Autodesk Inventor part; units mm, degrees
ref_plane "YZ Plane" through (0, 0, 0) normal (1, 0, 0) x (0, 1, 0)
ref_plane "XZ Plane" through (0, 0, 0) normal (0, 1, 0) x (-1, 0, 0)
ref_plane "XY Plane" through (0, 0, 0) normal (0, 0, 1) x (1, 0, 0)
sketch "스케치1" plane through (0, 0, 0) normal (0, 0, 1) x (1, 0, 0)
  circle A0 centre (-35.1217, 0) radius 22.9499
  circle A1 centre (-35.1217, 0) radius 11.4294
  line L0 (-20.9226, -18.03) -> (64.9173, -18.03)
  line L1 (64.9173, -18.03) -> (64.9173, 18.03)
  line L2 (64.9173, 18.03) -> (-20.9226, 18.03)
  point P0 (0, 0)
extrude "돌출1" add sketch "스케치1" along normal blind 30 contours A0 L2 L1 L0
extrude "돌출2" add sketch "스케치1" along normal blind 40 contours A0
sketch "스케치2" plane through (-35.1217, 0, 40) normal (0, 0, 1) x (1, 0, 0)
  circle A0 centre (0, 0) radius 11.4294
  line L0 (9.9823, 5.5664) -> (22.2646, 5.5664)
  circle A1 centre (0, 0) radius 22.9499
  line L1 (9.9823, -5.5664) -> (22.2646, -5.5664)
  line L2 (-9.9823, 5.5664) -> (-22.2646, 5.5664)
  line L3 (-9.9823, -5.5664) -> (-22.2646, -5.5664)
  point P0 (35.1217, 0)
extrude "돌출3" add sketch "스케치2" along normal blind 10 contours A0 L0 A1 L1 | A0 L3 A1 L2
sketch "스케치3" plane through (0, 0, 30) normal (0, 0, 1) x (1, 0, 0)
  line L0 (64.9173, -18.03) -> (64.9173, 18.03)
  line L1 (-5.4969, 10.1103) -> (64.9173, 10.1103)
  line L2 (64.9173, 10.1103) -> (64.9173, -11.6809)
  line L3 (64.9173, -11.6809) -> (-5.4969, -11.6809)
  line L4 (-5.4969, -11.6809) -> (-5.4969, 10.1103)
  circle A0 centre (15.1164, 0) radius 4.8497
  circle A1 centre (45.3492, 0) radius 4.9674
  point P0 (0, 0)
extrude "돌출4" cut sketch "스케치3" against normal blind 50 contours A0 | A1
extrude "돌출5" cut sketch "스케치3" against normal blind 20
chamfer "모따기1" distance 13 angle 45 2 edges at (64.9173, 14.0702, 30) (64.9173, -14.8554, 30)
properties part number "240510_3Dsketch06"
Source: CAD feature listing. Evaluate the final solid. Frame: model axes, mm. A direction names the side the tool comes from. Coordinates: 2 decimals unless noted, no trailing zeros. Write each loop counter-clockwise with the first axis right and the second up, starting at its lowest first coordinate (ties: lowest second). Pieces come first, ordered by that corner, then holes. Notation, with made-up numbers: (-17, 89) -> (8, 89) arc R23 ccw to (8, 118) -> close; hole circle Ø4 at (7.25, 46). An arc over 180 degrees is marked (long way). Return JSON: item names as keys, results as strings. Group by question number.
1) Mould query, pull axis Y, two halves, no side actions, for faces 1 (the face through (23, 18.03, 15)), 2 (the face through (-19, 0, 50)), 3 (the face through (-5.497, -1, 20)), 4 (the face through (-57.75, -3.84, 24.65)). Classes: +Y half, -Y half, draft (parallel to the pull), parting line (faces both ways), or undercut.
2) Contact query for flat-ended pins moving along their axis: P1, Ø3, axis at x = -21.5, z = 45, coming from the +Y side; P2, Ø8.5, axis at x = -36.5, y = 11, coming from the +Z side; P3, Ø15, axis at x = 24.5, z = 17.5, coming from the -Y side. Output: stop coordinate, or through.
3) Section query A-A, the plane y = -8. Return loops of the section in (x, z), plus the area to 3 significant figures.
4) Section query C-C, the plane y = -3. Return loops of the section in (x, z), plus the area to 3 significant figures.
5) Ray query, line 1 along Y through (x, z) = (4, 13.5); line 2 along Y through (x, z) = (-7, 23); line 3 along X through (y, z) = (4, 35.5). Return the intervals inside material, ascending.
6) Set-up query: faces 5 (the face through (58.33, 14.13, 23.59)), 6 (the face through (-51, -5.566, 45)), 7 (the face through (29, 10.11, 20)), 8 (the face through (-19, 5.566, 45)). Return all of +Z, -Z, +X, -X, +Y, -Y with unobstructed straight access to the full face (end or side cutting, diameter ignored); none if empty.
7) Section query B-B, the plane z = 8. Return loops of the section in (x, y).
8) Section query D-D, the plane x = 23. Return loops of the section in (y, z), plus the area to 3 significant figures.
From the geometry:
{
 "1": {"face 1": "+Y half", "face 2": "draft", "face 3": "undercut", "face 4": "parting line"},
 "2": {"P1": "y = 5.57", "P2": "z = 40", "P3": "y = -18.03"},
 "3": {"outline": "(-56.63, 0) -> (-43.28, 0) -> (-43.28, 40) -> (-56.63, 40) -> close; (-26.96, 0) -> (64.92, 0) -> (64.92, 10) -> (-5.5, 10) -> (-5.5, 30) -> (-13.61, 30) -> (-13.61, 40) -> (-26.96, 40) -> close", "area": "2,020 mm²"},
 "4": {"outline": "(-57.87, 0) -> (-46.15, 0) -> (-46.15, 50) -> (-57.87, 50) -> close; (-24.09, 0) -> (11.31, 0) -> (11.31, 10) -> (-5.5, 10) -> (-5.5, 30) -> (-12.37, 30) -> (-12.37, 50) -> (-24.09, 50) -> close; (18.93, 0) -> (41.39, 0) -> (41.39, 10) -> (18.93, 10) -> close; (49.31, 0) -> (64.92, 0) -> (64.92, 10) -> (49.31, 10) -> close", "area": "1,930 mm²"},
 "5": {"line 1": "-18.03 to -11.68, 10.11 to 18.03", "line 2": "-18.03 to 18.03", "line 3": "-57.72 to -45.83, -24.42 to -12.52"},
 "6": {"face 5": "+Z, +X, +Y, -Y", "face 6": "+Z, +X, -X, -Y", "face 7": "+Z, +X", "face 8": "+Z, +X, -X, +Y"},
 "7": {"outline": "(-20.92, -18.03) -> (64.92, -18.03) -> (64.92, 18.03) -> (-20.92, 18.03) arc R22.95 ccw (long way) to start; hole circle Ø22.86 at (-35.12, 0); hole circle Ø9.7 at (15.12, 0); hole circle Ø9.93 at (45.35, 0)"},
 "8": {"outline": "(-18.03, 0) -> (18.03, 0) -> (18.03, 30) -> (10.11, 30) -> (10.11, 10) -> (-11.68, 10) -> (-11.68, 30) -> (-18.03, 30) -> close", "area": "646 mm²"}
}
